The listing builds one solid part. Answer for the finished solid, in the listing's coordinates (mm). A direction names the side the tool comes from. Round coordinates to 2 decimals unless told otherwise and drop trailing zeros. Write each loop counter-clockwise with the first axis right and the second up, starting at its lowest first coordinate (ties: lowest second). Pieces come first, ordered by that corner, then holes. Notation, with made-up numbers: M -10.75,42 L 43.25,42 A22 ccw 43.25,79 Z; hole C 21,-14 d6. An arc over 180 degrees is marked long. Write each question's results on one line, items separated by ' | '.
from build123d import *

# Parameters (mm, degrees)
SKETCH_1_W          = 42
SKETCH_1_H          = 20
EXTRUDE_1_DEPTH     = 1
SKETCH_2_W          = 1
SKETCH_2_H          = 20
EXTRUDE_2_DEPTH     = 18
CUT_EXTRUDE_1_REACH = 49.17
SKETCH_3_R          = 0.5
FILLET_1_R          = 2
FILLET_2_R          = 2
FILLET_4_R          = 2
CUT_EXTRUDE_2_REACH = 49.17
SKETCH_6_R          = 0.5
SKETCH_7_R          = 1.5
CUT_EXTRUDE_3_DEPTH = 10


with BuildPart() as part:
    # 草图1 → 凸台-拉伸1 (new body)
    with BuildSketch(Plane.XY):
        Rectangle(SKETCH_1_W, SKETCH_1_H)
    extrude(amount=EXTRUDE_1_DEPTH)

    # 草图2 → 凸台-拉伸2 (add)
    with BuildSketch(Plane.XY.offset(1)):
        with Locations((-20.5, 0)):
            Rectangle(SKETCH_2_W, SKETCH_2_H)
        with Locations((20.5, 0)):
            Rectangle(SKETCH_2_W, SKETCH_2_H)
    extrude(amount=EXTRUDE_2_DEPTH)

    # 草图3 → 切除-拉伸1 (cut, up to next)
    with BuildSketch(Plane(origin=(21, 0, 0), x_dir=(0, 0, -1), z_dir=(1, 0, 0)), mode=Mode.PRIVATE) as cut_extrude_1_sk1:
        with Locations(Location((-17, 8, 0), (0, 0, 90))):
            Circle(SKETCH_3_R)
    cut_extrude_1_tool1 = extrude(cut_extrude_1_sk1.sketch, amount=-CUT_EXTRUDE_1_REACH, mode=Mode.PRIVATE) & part.part
    # 草图3 → 切除-拉伸1 (cut, up to next)
    with BuildSketch(Plane(origin=(21, 0, 0), x_dir=(0, 0, -1), z_dir=(1, 0, 0)), mode=Mode.PRIVATE) as cut_extrude_1_sk2:
        with Locations(Location((-7, 8, 0), (0, 0, 90))):
            Circle(SKETCH_3_R)
    cut_extrude_1_tool2 = extrude(cut_extrude_1_sk2.sketch, amount=-CUT_EXTRUDE_1_REACH, mode=Mode.PRIVATE) & part.part
    # 草图3 → 切除-拉伸1 (cut, up to next)
    with BuildSketch(Plane(origin=(21, 0, 0), x_dir=(0, 0, -1), z_dir=(1, 0, 0)), mode=Mode.PRIVATE) as cut_extrude_1_sk3:
        with Locations(Location((-7, -8, 0), (0, 0, 90))):
            Circle(SKETCH_3_R)
    cut_extrude_1_tool3 = extrude(cut_extrude_1_sk3.sketch, amount=-CUT_EXTRUDE_1_REACH, mode=Mode.PRIVATE) & part.part
    # 草图3 → 切除-拉伸1 (cut, up to next)
    with BuildSketch(Plane(origin=(21, 0, 0), x_dir=(0, 0, -1), z_dir=(1, 0, 0)), mode=Mode.PRIVATE) as cut_extrude_1_sk4:
        with Locations(Location((-17, -8, 0), (0, 0, 90))):
            Circle(SKETCH_3_R)
    cut_extrude_1_tool4 = extrude(cut_extrude_1_sk4.sketch, amount=-CUT_EXTRUDE_1_REACH, mode=Mode.PRIVATE) & part.part
    add(cut_extrude_1_tool1.solids().sort_by_distance((21, 8, 17))[0], mode=Mode.SUBTRACT)
    add(cut_extrude_1_tool2.solids().sort_by_distance((21, 8, 7))[0], mode=Mode.SUBTRACT)
    add(cut_extrude_1_tool3.solids().sort_by_distance((21, -8, 7))[0], mode=Mode.SUBTRACT)
    add(cut_extrude_1_tool4.solids().sort_by_distance((21, -8, 17))[0], mode=Mode.SUBTRACT)

    # 圆角1
    fillet_1_edges = [part.edges().sort_by_distance(p)[0] for p in [
        (20.5, 10, 19),
        (20.5, -10, 19),
    ]]
    fillet(fillet_1_edges, radius=FILLET_1_R)

    # 圆角2
    fillet_2_edges = [part.edges().sort_by_distance(p)[0] for p in [
        (-20.5, 10, 19),
    ]]
    fillet(fillet_2_edges, radius=FILLET_2_R)

    # 圆角4
    fillet_4_edges = [part.edges().sort_by_distance(p)[0] for p in [
        (-20.5, -10, 19),
    ]]
    fillet(fillet_4_edges, radius=FILLET_4_R)

    # 草图6 → 切除-拉伸2 (cut, up to next)
    with BuildSketch(Plane.ZY.offset(21), mode=Mode.PRIVATE) as cut_extrude_2_sk1:
        with Locations((12, 0)):
            Circle(SKETCH_6_R)
    cut_extrude_2_tool1 = extrude(cut_extrude_2_sk1.sketch, amount=-CUT_EXTRUDE_2_REACH, mode=Mode.PRIVATE) & part.part
    add(cut_extrude_2_tool1.solids().sort_by_distance((-21, 0, 12))[0], mode=Mode.SUBTRACT)

    # 草图7 → 切除-拉伸3 (cut)
    with BuildSketch(Plane(origin=(0, 0, 0), x_dir=(-1, 0, 0), z_dir=(0, 0, -1))):
        with Locations((5, -5)):
            Circle(SKETCH_7_R)
        with Locations((-5, -5)):
            Circle(SKETCH_7_R)
        with Locations((-5, 5)):
            Circle(SKETCH_7_R)
        with Locations((5, 5)):
            Circle(SKETCH_7_R)
    extrude(amount=-CUT_EXTRUDE_3_DEPTH, mode=Mode.SUBTRACT)


solid = part.part
1) The mould has two halves that part along Y. Classify faces 6 (the face through (20.5, 0.1, 19)), 7 (the face through (-20.49, 9.43, 18.4)), 8 (the face through (20.507, 8.231, 6.556)): +Y half, -Y half, draft (parallel to the pull), parting line (faces both ways), or undercut.
Return value:
face 6: draft | face 7: +Y half | face 8: undercut
2) Find the intervals of material crossed by line 1 (Y direction, x = -5, z = 0.7); line 2 (X direction, y = 8.75, z = 4); line 3 (Y direction, x = -20.6, z = 12), in increasing order.
Return value:
line 1: -10 to -6.5, -3.5 to 3.5, 6.5 to 10 | line 2: -21 to -20, 20 to 21 | line 3: -10 to -0.5, 0.5 to 10
3) A tool of negligible diameter and unlimited length cuts with its end or side. For faces 1 (the face through (20.5, -7.7, 17.4)), 2 (the face through (0, 0, 0)), 3 (the face through (0, 0, 1)), 4 (the face through (20.51, 9.43, 18.4)), 5 (the face through (-20.5, 0, 11.5)), from which of +Z, -Z, +X, -X, +Y, -Y can it reach the whole face along a straight path? Write none if from no direction.
Return value:
face 1: +X | face 2: -Z, +X, -X, +Y, -Y | face 3: +Z, +Y, -Y | face 4: +Z, +X, -X, +Y | face 5: -X
4) Section B-B (z = 7) is taken. Determine the outline of the cut face in (x, y).
Return value:
outline: M -21,-10 L -20,-10 L -20,10 L -21,10 Z; M 20,-10 L 21,-10 L 21,-8.5 L 20,-8.5 Z; M 20,-7.5 L 21,-7.5 L 21,7.5 L 20,7.5 Z; M 20,8.5 L 21,8.5 L 21,10 L 20,10 Z
5) Section D-D (z = 13) is taken. Determine the outline of the cut face in (x, y), then the cut area to 3 significant figures.
Return value:
outline: M -21,-10 L -20,-10 L -20,10 L -21,10 Z; M 20,-10 L 21,-10 L 21,10 L 20,10 Z | area: 40.0 mm²
6) Section C-C (y = -5) is taken. Determine the outline of the cut face in (x, z).
Return value:
outline: M -21,0 L -6.5,0 L -6.5,1 L -20,1 L -20,19 L -21,19 Z; M -3.5,0 L 3.5,0 L 3.5,1 L -3.5,1 Z; M 6.5,0 L 21,0 L 21,19 L 20,19 L 20,1 L 6.5,1 Z
7) This flat-tipped pin is pushed along its axis until it touches: pin 1 (6 mm diameter, centred on x = -0.5, y = 0.5, fed in from +Z). Where does it stop, or does it pass through?
Return value:
pin 1: z = 1
8) Section A-A (y = 0) is taken. Determine the outline of the cut face in (x, z).
Return value:
outline: M -21,0 L 21,0 L 21,19 L 20,19 L 20,1 L -20,1 L -20,11.5 L -21,11.5 Z; M -21,12.5 L -20,12.5 L -20,19 L -21,19 Z
